Build history of the part. All positions in model axes, mm. Coordinates: 2 decimals unless noted, no trailing zeros. Order: outer loops, then holes, each group sorted by start corner. A loop starts at its lowest first (then second) coordinate and runs counter-clockwise, first axis right, second up. Notation, with made-up numbers: (0, 50.25) - (18, 50.25) arc R25 ccw to (18, 78.25) - close; hole circle Ø8 at (4.25, 19.5). An arc over 180 degrees is marked (long way). Write each question's results on one line, items separated by ' | '. Start each with the question number.
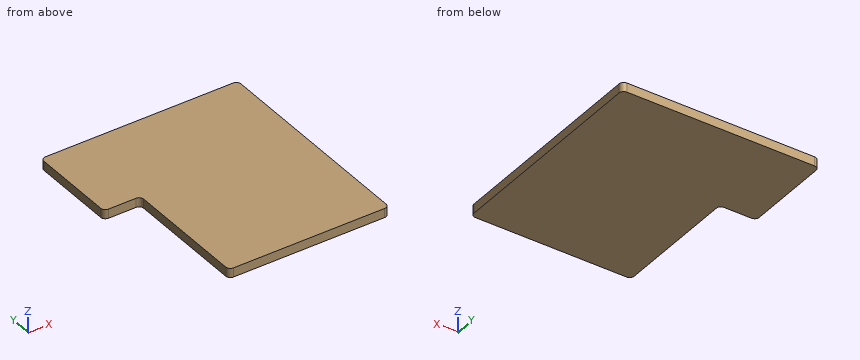
from build123d import *

# Parameters (mm, degrees)
EXTRUDE_1_DEPTH = 1


with BuildPart() as part:
    # 草图1 → 凸台-拉伸1 (new body)
    with BuildSketch(Plane.XY):
        with BuildLine():
            Line((1.5, 24), (-3.5, 24))
            ThreePointArc((-3.5, 24), (-3.853553391, 23.853553391), (-4, 23.5))
            Line((-4, 23.5), (-4, 14.5))
            ThreePointArc((-4, 14.5), (-3.853553391, 14.146446609), (-3.5, 14))
            Line((-3.5, 14), (-0.5, 14))
            ThreePointArc((-0.5, 14), (-0.146446609, 13.853553391), (0, 13.5))
            Line((0, 13.5), (0, 0.5))
            ThreePointArc((0, 0.5), (0.146446609, 0.146446609), (0.5, 0))
            Line((0.5, 0), (17, 0))
            ThreePointArc((17, 0), (17.353553391, 0.146446609), (17.5, 0.5))
            Line((17.5, 0.5), (17.5, 23.5))
            ThreePointArc((17.5, 23.5), (17.353553391, 23.853553391), (17, 24))
            Line((17, 24), (1.5, 24))
        make_face()
    extrude(amount=EXTRUDE_1_DEPTH)


solid = part.part
Item 1: Slice it at B-B (y = 12.75). Write the cut outline in (x, z), then the cut area to 3 significant figures.
Item 2: Slice it at A-A (z = 0.4). Write the cut outline in (x, y).
Item 3: Probe probe 1 along X at (y, z) = (11.75, 0.4); probe 2 along Y at (x, z) = (-0.5, 0.8). List the from-to ranges inside material, lowest first.
Item 4: Slice it at C-C (x = -1.5). Write the cut outline in (y, z), then the cut area to 4 significant figures.
Resolved:
1) outline: (0, 0) - (17.5, 0) - (17.5, 1) - (0, 1) - close | area: 17.5 mm^2
2) outline: (-4, 14.5) arc R0.5 ccw to (-3.5, 14) - (-0.5, 14) arc R0.5 cw to (0, 13.5) - (0, 0.5) arc R0.5 ccw to (0.5, 0) - (17, 0) arc R0.5 ccw to (17.5, 0.5) - (17.5, 23.5) arc R0.5 ccw to (17, 24) - (-3.5, 24) arc R0.5 ccw to (-4, 23.5) - close
3) probe 1: 0 to 17.5 | probe 2: 14 to 24
4) outline: (14, 0) - (24, 0) - (24, 1) - (14, 1) - close | area: 10.00 mm^2
